```python
from build123d import *

# Parameters (mm, degrees)
SKETCH1_R           = 5.715
BOSS_EXTRUDE1_DEPTH = 9.525
SKETCH2_R           = 4.0132
BOSS_EXTRUDE2_DEPTH = 3.175
SKETCH3_R           = 5.715
BOSS_EXTRUDE3_DEPTH = 0.889
SKETCH4_R           = 3.175
CUT_EXTRUDE1_DEPTH  = 16.810862437
SKETCH5_R           = 4.0386
CUT_EXTRUDE2_DEPTH  = 8.255


with BuildPart() as part:
    # Sketch1 → Boss-Extrude1 (new body)
    with BuildSketch(Plane(origin=(0, 0, 0), x_dir=(0, 0, -1), z_dir=(1, 0, 0))):
        with Locations(Location((0, 0, 0), (0, 0, 180))):
            Circle(SKETCH1_R)
    extrude(amount=BOSS_EXTRUDE1_DEPTH)

    # Sketch2 → Boss-Extrude2 (add)
    with BuildSketch(Plane(origin=(9.525, 0, 0), x_dir=(0, 0, -1), z_dir=(1, 0, 0))):
        Circle(SKETCH2_R)
    extrude(amount=BOSS_EXTRUDE2_DEPTH)

    # Sketch3 → Boss-Extrude3 (add)
    with BuildSketch(Plane(origin=(12.7, 0, 0), x_dir=(0, 0, -1), z_dir=(1, 0, 0))):
        with Locations(Location((0, 0, 0), (0, 0, 180))):
            Circle(SKETCH3_R)
    extrude(amount=BOSS_EXTRUDE3_DEPTH)

    # Sketch4 → Cut-Extrude1 (cut, through all)
    with BuildSketch(Plane(origin=(13.589, 0, 0), x_dir=(0, 0, -1), z_dir=(1, 0, 0))):
        Circle(SKETCH4_R)
    extrude(amount=-CUT_EXTRUDE1_DEPTH, mode=Mode.SUBTRACT)

    # Sketch5 → Cut-Extrude2 (cut)
    with BuildSketch(Plane.ZY):
        Circle(SKETCH5_R)
    extrude(amount=-CUT_EXTRUDE2_DEPTH, mode=Mode.SUBTRACT)


solid = part.part
```
Verification items for the finished model (mm, model axes). A direction names the side the tool comes from. Give positions to 0.01 mm unless a question says otherwise; leave off trailing zeros. Loops run counter-clockwise (first coordinate to the right, second up) from the corner with the lowest first, then second, coordinate; pieces in that order, holes last.
1. Go/stop test with flat-tipped pins: pin 1 Ø5.5 at (y, z) = (3, -2.5) entering from -X; pin 2 Ø4 at (x, z) = (11.5, 3) entering from +Y; pin 3 Ø4 at (x, z) = (3.5, -2.5) entering from +Y; pin 4 Ø1.5 at (x, z) = (9.5, 3.5) entering from +Y. Record where each tip stops, or that it passes through.
2. Mould release check, pull along Y, two halves, no side actions. Record for faces 4 (the cylindrical face through (11.09, 2.71, 2.96)), 5 (the cylindrical face through (10.96, -3.1, 0.69)), 6 (the flat face through (0, 4, 2)), 7 (the flat face through (8.255, -3, 2)): released by +Y, released by -Y, zero draft, split by the parting line, or undercut.
3. Set-up check for faces 1 (the flat face through (12.7, 4, 2)), 2 (the cylindrical face through (4.696, 3.477, -4.535)), 3 (the cylindrical face through (4.07, 1.213, 3.852)): record each of +Z, -Z, +X, -X, +Y, -Y from which the full face is reachable in a straight line by a thin tool's end or side.
4. Section check D-D, the plane x = 8.5. Enter the section's corners in (y, z) (3 decimals), then the cut area to 3 significant figures.
5. Thickness scan on line 1 (X direction, y = -1.75, z = -5) (3 decimals); line 2 (Y direction, x = 11, z = 0) (3 decimals); line 3 (Y direction, x = 6, z = 0) (3 decimals). Record the ranges inside material, lowest first.
6. Section check C-C, the plane x = 5.25. Enter the section's corners in (y, z) (3 decimals), then the cut area to 3 significant figures.
7. Section check A-A, the plane z = 0. Enter the section's corners in (x, y) (3 decimals).
Geometry says:
1. pin 1: stops at x = 0
1. pin 2: stops at y = 5.54
1. pin 3: stops at y = 5.69
1. pin 4: stops at y = 5.01
2. face 4: split by the parting line
2. face 5: undercut
2. face 6: zero draft
2. face 7: undercut
3. face 1: none
3. face 2: +X, -X
3. face 3: -X
4. outline: circle Ø11.43 at (0, 0); hole circle Ø6.35 at (0, 0)
4. area: 70.9 mm2
5. line 1: x = 0 to 9.525, 12.7 to 13.589
5. line 2: y = -4.013 to -3.175, 3.175 to 4.013
5. line 3: y = -5.715 to -4.039, 4.039 to 5.715
6. outline: circle Ø11.43 at (0, 0); hole circle Ø8.077 at (0, 0)
6. area: 51.4 mm2
7. outline: (0, -5.715) - (9.525, -5.715) - (9.525, -4.013) - (12.7, -4.013) - (12.7, -5.715) - (13.589, -5.715) - (13.589, -3.175) - (8.255, -3.175) - (8.255, -4.039) - (0, -4.039) - close; (0, 4.039) - (8.255, 4.039) - (8.255, 3.175) - (13.589, 3.175) - (13.589, 5.715) - (12.7, 5.715) - (12.7, 4.013) - (9.525, 4.013) - (9.525, 5.715) - (0, 5.715) - close
